from build123d import *

# Parameters (mm, degrees)
SZKIC1_R                         = 12
DODANIE_WYCI_GNI_CIE6_DEPTH      = 17
DODANIE_WYCI_GNI_CIE6_DEPTH_BACK = 17


with BuildPart() as part:
    # Szkic1 → Dodanie-wyci_gni_cie6 (new body, two sides)
    with BuildSketch(Plane.XY) as dodanie_wyci_gni_cie6_sk:
        with BuildLine():
            ThreePointArc((30.970807503, 10.515463918), (25.991622783, -1.505351363), (13.970807503, -6.484536082))
            Line((13.970807503, -6.484536082), (4.970807503, -6.484536082))
            Line((4.970807503, -6.484536082), (-43.029192497, -6.484536082))
            Line((-43.029192497, -6.484536082), (-43.029192497, 27.515463918))
            Line((-43.029192497, 27.515463918), (4.970807503, 27.515463918))
            Line((4.970807503, 27.515463918), (13.970807503, 27.515463918))
            ThreePointArc((13.970807503, 27.515463918), (25.991622783, 22.536279198), (30.970807503, 10.515463918))
        make_face()
        with Locations((4.970807503, 10.515463918)):
            Circle(SZKIC1_R, mode=Mode.SUBTRACT)
    extrude(amount=DODANIE_WYCI_GNI_CIE6_DEPTH)
    extrude(dodanie_wyci_gni_cie6_sk.sketch, amount=-DODANIE_WYCI_GNI_CIE6_DEPTH_BACK)


solid = part.part
Read the model definition and answer for the solid it produces. Units are mm, in the model's axes. Round coordinates to 2 decimals unless told otherwise and drop trailing zeros. Write each loop counter-clockwise with the first axis right and the second up, starting at its lowest first coordinate (ties: lowest second). Pieces come first, ordered by that corner, then holes. Notation, with made-up numbers: M -8.75,69.5 L 34.25,69.5 A11 cw 34.25,75.5 Z; hole C 7,25.5 d7. An arc over 180 degrees is marked long. Use a Markdown table: item, result.
1) The part is cut by section D-D (y = -3). Write down the section's boundary in (x, z).
Answers follow:
| item | result |
|---|---|
| outline | M -43.03,-17 L 24.28,-17 L 24.28,17 L -43.03,17 Z |
2) The part is cut by section A-A (x = 9). Write down the section's boundary in (y, z), plus the area to 3 significant figures.
Answers follow:
| item | result |
|---|---|
| outline | M -6.48,-17 L -0.79,-17 L -0.79,17 L -6.48,17 Z; M 21.82,-17 L 27.52,-17 L 27.52,17 L 21.82,17 Z |
| area | 387 mm2 |
3) Straight lines are drawn through the part: line 1 along X through (y, z) = (11, -15); line 2 along X through (y, z) = (12, 15); line 3 along Y through (x, z) = (9.5, -1.5). For each, find the intervals that lie inside material, in ascending order. Write a range as [from, to].
Answers follow:
| item | result |
|---|---|
| line 1 | x = [-43.03, -7.02], [16.96, 30.96] |
| line 2 | x = [-43.03, -6.94], [16.88, 30.91] |
| line 3 | y = [-6.48, -0.6], [21.63, 27.52] |
4) Flat-ended cylindrical pins translate along their axes: pin 1 (14.5 mm diameter, centred on x = 4.97, y = 10.52, fed in from +Z); pin 2 (8 mm diameter, centred on y = 20, z = 11, fed in from +X). Find the tip coordinate at first contact, or state that the pin passes through.
Answers follow:
| item | result |
|---|---|
| pin 1 | passes through |
| pin 2 | stops at x = 30.06 |
5) The part is cut by section B-B (y = 6). Write down the section's boundary in (x, z).
Answers follow:
| item | result |
|---|---|
| outline | M -43.03,-17 L -6.15,-17 L -6.15,17 L -43.03,17 Z; M 16.09,-17 L 30.36,-17 L 30.36,17 L 16.09,17 Z |
6) The part is cut by section C-C (z = 5.5). Write down the section's boundary in (x, y), plus the area to 3 significant figures.
Answers follow:
| item | result |
|---|---|
| outline | M -43.03,-6.48 L 13.97,-6.48 A17 ccw 13.97,27.52 L -43.03,27.52 Z; hole C 4.97,10.52 d24 |
| area | 1,940 mm2 |
